from build123d import *

# Parameters (mm, degrees)
BOSS_EXTRUDE2_DEPTH       = 6
BOSS_EXTRUDE3_DEPTH       = 24
BOSS_EXTRUDE5_START       = 12
SKETCH7_R                 = 24
BOSS_EXTRUDE5_DEPTH       = 56
BOSS_EXTRUDE6_START       = 4
SKETCH4_W                 = 16
SKETCH4_H                 = 56
BOSS_EXTRUDE6_DEPTH       = 56
M24_CLEARANCE_SLOT4_D     = 24
M24_CLEARANCE_SLOT4_DEPTH = 56


with BuildPart() as part:
    # Sketch1 → Boss-Extrude2 (new, symmetric)
    with BuildSketch(Plane(origin=(0, 0, 0), x_dir=(1, 0, 0), z_dir=(0, 1, 0))):
        with BuildLine():
            ThreePointArc((12, 0), (18.202041029, -12.649110641), (32, -15.491933385))
            Line((32, -15.491933385), (32, 0))
            Line((32, 0), (32, 72))
            ThreePointArc((32, 72), (37.857864376, 86.142135624), (52, 92))
            Line((52, 92), (168, 92))
            ThreePointArc((168, 92), (182.142135624, 86.142135624), (188, 72))
            Line((188, 72), (188, 0))
            Line((188, 0), (208, 0))
            Line((208, 0), (208, 108))
            ThreePointArc((208, 108), (202.142135624, 122.142135624), (188, 128))
            Line((188, 128), (32, 128))
            ThreePointArc((32, 128), (17.857864376, 122.142135624), (12, 108))
            Line((12, 108), (12, 0))
        make_face()
    extrude(amount=BOSS_EXTRUDE2_DEPTH, both=True)

    # Sketch1<4> → Boss-Extrude3 (add, symmetric)
    with BuildSketch(Plane(origin=(0, 0, 0), x_dir=(1, 0, 0), z_dir=(0, 1, 0))):
        with BuildLine():
            Line((0, 108), (0, 0))
            ThreePointArc((0, 0), (9.66969722, -21.166010489), (32, -27.712812921))
            Line((32, -27.712812921), (32, -15.491933385))
            ThreePointArc((32, -15.491933385), (18.202041029, -12.649110641), (12, 0))
            Line((12, 0), (12, 108))
            ThreePointArc((12, 108), (17.857864376, 122.142135624), (32, 128))
            Line((32, 128), (188, 128))
            ThreePointArc((188, 128), (202.142135624, 122.142135624), (208, 108))
            Line((208, 108), (208, 0))
            Line((208, 0), (220, 0))
            Line((220, 0), (220, 108))
            ThreePointArc((220, 108), (210.627416998, 130.627416998), (188, 140))
            Line((188, 140), (32, 140))
            ThreePointArc((32, 140), (9.372583002, 130.627416998), (0, 108))
        make_face()
        with BuildLine():
            Line((32, 72), (32, 0))
            Line((32, 0), (44, 0))
            Line((44, 0), (44, 72))
            ThreePointArc((44, 72), (46.343145751, 77.656854249), (52, 80))
            Line((52, 80), (168, 80))
            ThreePointArc((168, 80), (173.656854249, 77.656854249), (176, 72))
            Line((176, 72), (176, 0))
            Line((176, 0), (188, 0))
            Line((188, 0), (188, 72))
            ThreePointArc((188, 72), (182.142135624, 86.142135624), (168, 92))
            Line((168, 92), (52, 92))
            ThreePointArc((52, 92), (37.857864376, 86.142135624), (32, 72))
        make_face()
    extrude(amount=BOSS_EXTRUDE3_DEPTH, both=True)

    # Sketch7 → Boss-Extrude5 (add)
    with BuildSketch(Plane(origin=(220, 0, 0), x_dir=(0, 0, -1), z_dir=(1, 0, 0)).offset(BOSS_EXTRUDE5_START)):
        Circle(SKETCH7_R)
    extrude(amount=-BOSS_EXTRUDE5_DEPTH)

    # Sketch4 → Boss-Extrude6 (add)
    with BuildSketch(Plane(origin=(0, 24, 0), x_dir=(1, 0, 0), z_dir=(0, 1, 0)).offset(BOSS_EXTRUDE6_START)):
        with Locations((40, 0.287187079)):
            Rectangle(SKETCH4_W, SKETCH4_H)
    extrude(amount=-BOSS_EXTRUDE6_DEPTH)

    # M24 Clearance Slot4
    with Locations(Plane(origin=(232, 0, 0), x_dir=(0, 0, -1), z_dir=(1, 0, 0))):
        with Locations((0, 0)):
            Hole(M24_CLEARANCE_SLOT4_D / 2, depth=M24_CLEARANCE_SLOT4_DEPTH)


solid = part.part
Work out the finished part from the listing and answer in its coordinate system (mm). A direction names the side the tool comes from. Coordinates: 2 decimals unless noted, no trailing zeros. Loops run counter-clockwise (first coordinate to the right, second up) from the corner with the lowest first, then second, coordinate; pieces in that order, holes last. Notation, with made-up numbers: M -5.75,78.5 L 26.25,78.5 A28 ccw 26.25,112.5 Z; hole C -17,-7.75 d5. An arc over 180 degrees is marked long. Answer in a Markdown table with one row per item. Add a question column.
1. The mould has two halves that part along Z. Classify faces 1 (the flat face through (220, 0, -65)), 2 (the flat face through (188, -15, -43)), 3 (the cylindrical face through (9.62, -0.34, -130.87)): pulls with the +Z half, pulls with the -Z half, needs draft (parallel to the pull), parting line crosses it, or undercut.
2. Find section B-B, the plane z = -60. Write down the section's boundary in (x, y).
3. Find section C-C, the plane x = 199.5. Write down the section's boundary in (y, z), then the cut area to 3 significant figures.
4. Flat-ended cylindrical pins translate along their axes: P1, Ø14.5, axis at y = -13.5, z = -35, coming from the +X side; P2, Ø24, axis at x = 100.5, y = 11.5, coming from the +Z side; P3, Ø12, axis at x = 84, z = -102.5, coming from the +Y side. Find the tip coordinate at first contact, or state that the pin passes through.
5. A tool of negligible diameter and unlimited length cuts with its end or side. For faces 4 (the cylindrical face through (182.297, -14.874, -85.986)), 5 (the cylindrical face through (204.392, 1.055, 23.977)), 6 (the flat face through (208, 15, -67)), 7 (the flat face through (48, 0, 0)), from which of +Z, -Z, +X, -X, +Y, -Y can it reach the whole face along a straight path? Write none if from no direction.
6. Find section A-A, the plane y = 0. Write down the section's boundary in (x, z).
7. Find section D-D, the plane z = -100.5. Write down the section's boundary in (x, y), then the cut area to 3 significant figures.
8. Consider L1, parallel to X at y = -19, z = -53.5; L2, parallel to Z at x = 119, y = 20; L3, parallel to X at y = 9.5, z = -94. Determine where each line is inside the solid, lowest interval first.
Reported:
| question | item | result |
|---|---|---|
| 1 | face 1 | needs draft |
| 1 | face 2 | undercut |
| 1 | face 3 | pulls with the -Z half |
| 2 | outline | M 0,-24 L 12,-24 L 12,-6 L 32,-6 L 32,-24 L 44,-24 L 44,24 L 32,24 L 32,6 L 12,6 L 12,24 L 0,24 Z; M 176,-24 L 188,-24 L 188,-6 L 208,-6 L 208,-24 L 220,-24 L 220,24 L 208,24 L 208,6 L 188,6 L 188,24 L 176,24 Z |
| 3 | outline | M -24,-137.86 L 24,-137.86 L 24,-124.36 L 6,-124.36 L 6,-23.24 A24 ccw long -6,-23.24 L -6,-124.36 L -24,-124.36 Z; hole C 0,0 d24 |
| 3 | area | 3,210 mm^2 |
| 4 | P1 | stops at x = 220 |
| 4 | P2 | stops at z = -80 |
| 4 | P3 | stops at y = 6 |
| 5 | face 4 | -Y |
| 5 | face 5 | none |
| 5 | face 6 | +Y |
| 5 | face 7 | +Z, +Y, -Y |
| 6 | outline | M 0,-108 A32 ccw 32,-140 L 188,-140 A32 ccw 220,-108 L 220,-24 L 232,-24 L 232,-12 L 176,-12 L 176,-72 A8 cw 168,-80 L 52,-80 A8 cw 44,-72 L 44,-28.29 L 48,-28.29 L 48,27.71 L 32,27.71 A28 ccw 0,0 Z; M 176,12 L 232,12 L 232,24 L 176,24 Z |
| 7 | outline | M 0,-24 L 12,-24 L 12,-6 L 208,-6 L 208,-24 L 220,-24 L 220,24 L 208,24 L 208,6 L 12,6 L 12,24 L 0,24 Z |
| 7 | area | 3,500 mm^2 |
| 8 | L1 | x = 0 to 12, 32 to 44, 176 to 188, 208 to 220 |
| 8 | L2 | z = -140 to -128, -92 to -80 |
| 8 | L3 | x = 0 to 12, 208 to 220 |
